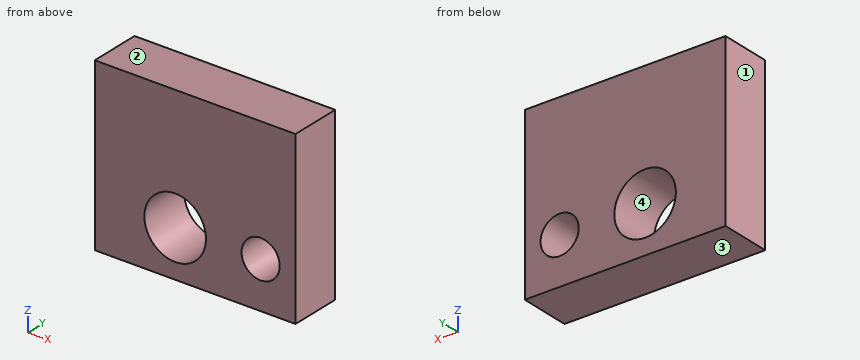
from build123d import *

# Parameters (mm, degrees)
F0_W     = 45.491502
F0_H     = 38.61044
F1_DEPTH = 11.6
F2_R     = 6.976475
F2_R_2   = 4.325021
F3_DEPTH = 25


with BuildPart() as f1:
    # F0 (on Front) → F1 (new body)
    with BuildSketch(Plane.XZ):
        with Locations((22.745751, 19.30522)):
            Rectangle(F0_W, F0_H)
    extrude(amount=F1_DEPTH)

    # F2 (on face) → F3 (cut)
    with BuildSketch(Plane(origin=(0, 0, 0), x_dir=(-1, 0, 0), z_dir=(0, 1, 0))):
        with Locations((-18.222088, 10.576457)):
            Circle(F2_R)
        with Locations((-37.591022, 10.576457)):
            Circle(F2_R_2)
    extrude(amount=-F3_DEPTH, mode=Mode.SUBTRACT)


solid = f1.part
Design review of the part built by this model. Coordinates are the model's own, in mm. Face numbers are marked on the shaded views. Coordinates: 2 decimals unless noted, no trailing zeros. Order: outer loops, then holes, each group sorted by start corner. A loop starts at its lowest first (then second) coordinate and runs counter-clockwise, first axis right, second up. Notation, with made-up numbers: M -34,-14 L -26,-14 A14 cw -26,-4 Z; hole C 46,49.5 d1. An arc over 180 degrees is marked long. Use a Markdown table: item, result.
(1) Add section D-D (y = -9). Give the boundary of the cut face in (x, z), then the cut area to 3 significant figures.
Worked answers:
| item | result |
|---|---|
| outline | M 0,0 L 45.49,0 L 45.49,38.61 L 0,38.61 Z; hole C 18.22,10.58 d13.95; hole C 37.59,10.58 d8.65 |
| area | 1,540 mm2 |
(2) Add section C-C (z = 12.5). Give the boundary of the cut face in (x, y).
Worked answers:
| item | result |
|---|---|
| outline | M 0,-11.6 L 11.52,-11.6 L 11.52,0 L 0,0 Z; M 24.93,-11.6 L 33.72,-11.6 L 33.72,0 L 24.93,0 Z; M 41.46,-11.6 L 45.49,-11.6 L 45.49,0 L 41.46,0 Z |
(3) Add section A-A (x = 14.5). Give the boundary of the cut face in (y, z).
Worked answers:
| item | result |
|---|---|
| outline | M -11.6,0 L 0,0 L 0,4.68 L -11.6,4.68 Z; M -11.6,16.48 L 0,16.48 L 0,38.61 L -11.6,38.61 Z |
(4) Add section B-B (z = 4.5). Give the boundary of the cut face in (x, y), then the cut area to 3 significant figures.
Worked answers:
| item | result |
|---|---|
| outline | M 0,-11.6 L 14.79,-11.6 L 14.79,0 L 0,0 Z; M 21.65,-11.6 L 45.49,-11.6 L 45.49,0 L 21.65,0 Z |
| area | 448 mm2 |
(5) Draft analysis for pull direction Z (two halves, no side actions). For the marked faces 1, 2, 3 and 4, state which applies: released by +Z, released by -Z, zero draft, split by the parting line, or undercut.
Worked answers:
| item | result |
|---|---|
| face 1 | zero draft |
| face 2 | released by +Z |
| face 3 | released by -Z |
| face 4 | undercut |
(6) Wall thickness on probe 1 along X at (y, z) = (-8, 8.5); probe 2 along Z at (x, y) = (18, -3.75); probe 3 along Z at (x, y) = (34.5, -2.25): over which ranges is each line inside the solid? List them lowest first.
Worked answers:
| item | result |
|---|---|
| probe 1 | x = 0 to 11.56, 24.88 to 33.8, 41.38 to 45.49 |
| probe 2 | z = 0 to 3.6, 17.55 to 38.61 |
| probe 3 | z = 0 to 7.55, 13.6 to 38.61 |
